Drawing for the job (mm, zero at the part's lowest x, y, z). Coordinates: 2 decimals unless noted, no trailing zeros. Write each loop counter-clockwise with the first axis right and the second up, starting at its lowest first coordinate (ties: lowest second). Pieces come first, ordered by that corner, then holes. Notation, with made-up numbers: (-34, 87.5) - (-2, 87.5) arc R21 ccw to (-2, 126.5) - close; hole circle Ø11 at (57, -27.75). An arc over 180 degrees is marked (long way). Write each question's results on one line, items separated by ' | '.
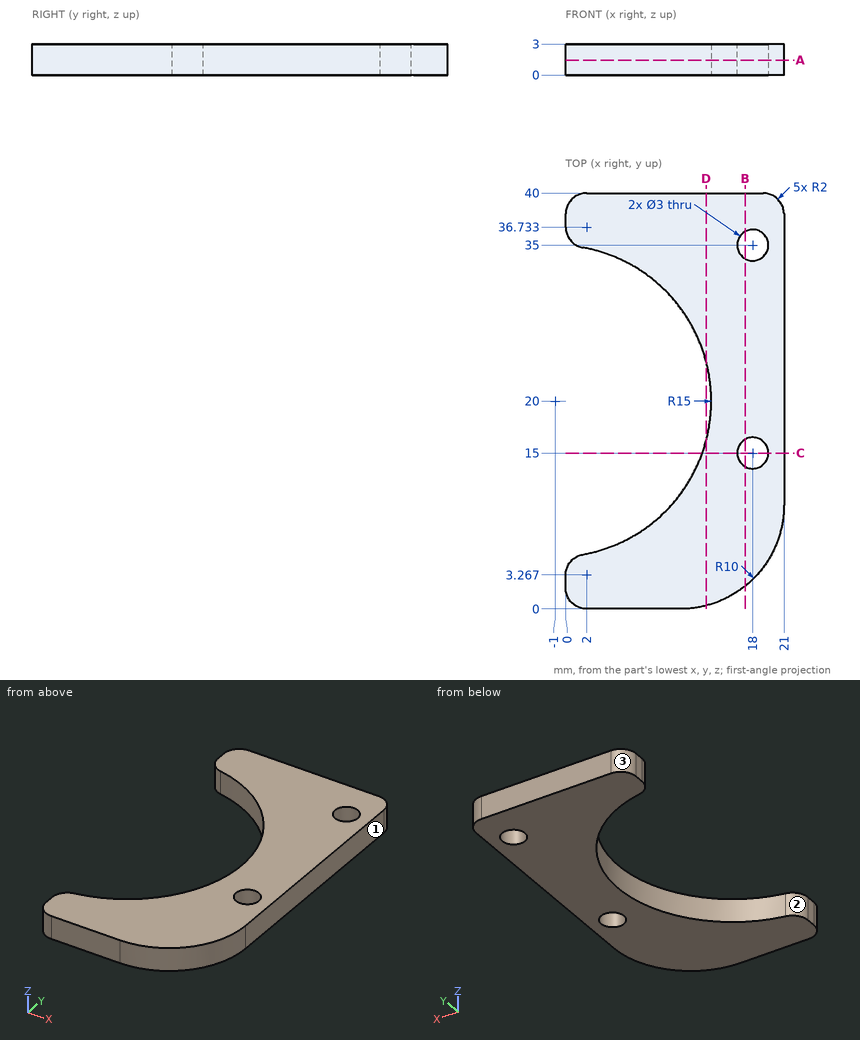
(1) Saw through at B-B on x = 17.25. Write the cut outline in (y, z).
Return value:
outline: (2.19, 0) - (13.7, 0) - (13.7, 3) - (2.19, 3) - close; (16.3, 0) - (33.7, 0) - (33.7, 3) - (16.3, 3) - close; (36.3, 0) - (40, 0) - (40, 3) - (36.3, 3) - close
(2) Flat gauge pins, fed straight in: P1, Ø2.5, axis at x = 18, y = 35, coming from the -Z side; P2, Ø1.5, axis at x = 14.5, z = 1, coming from the -Y side. Where does each tip first touch, or does it go through?
Return value:
P1: passes through | P2: stops at y = 0.39
(3) Wall check: line 1 (Y direction, x = 18, z = 1); line 2 (Y direction, x = 17, z = 0.95); line 3 (Y direction, x = 8.25, z = 2). Give the ranges that are in metal, low to high. Write a range as from..to.
Return value:
line 1: y = 2.86..13.5, 16.5..33.5, 36.5..40 | line 2: y = 2..13.88, 16.12..33.88, 36.12..40 | line 3: y = 0..8.19, 31.81..40
(4) Two-plate mould, pull along Y, no slides. Class the marked faces 1, 2 and 3: released by +Y, released by -Y, zero draft, split by the parting line, or undercut.
Return value:
face 1: zero draft | face 2: undercut | face 3: released by +Y
(5) Saw through at D-D on x = 13.5. Write the cut outline in (y, z), then the cut area to 3 significant figures.
Return value:
outline: (0.32, 0) - (16.16, 0) - (16.16, 3) - (0.32, 3) - close; (23.84, 0) - (40, 0) - (40, 3) - (23.84, 3) - close | area: 96.0 mm^2
(6) Saw through at C-C on y = 15. Write the cut outline in (x, z).
Return value:
outline: (13.14, 0) - (16.5, 0) - (16.5, 3) - (13.14, 3) - close; (19.5, 0) - (21, 0) - (21, 3) - (19.5, 3) - close
(7) Saw through at A-A on z = 1.45. Write the cut outline in (x, y), then the cut area to 3 significant figures.
Return value:
outline: (0, 2) arc R2 ccw to (2, 0) - (11, 0) arc R10 ccw to (21, 10) - (21, 38) arc R2 ccw to (19, 40) - (2, 40) arc R2 ccw to (0, 38) - (0, 36.73) arc R2 ccw to (1.65, 34.76) arc R15 cw to (1.65, 5.24) arc R2 ccw to (0, 3.27) - close; hole circle Ø3 at (18, 15); hole circle Ø3 at (18, 35) | area: 477 mm^2
